Verification items for the finished model (mm, model axes). A direction names the side the tool comes from. Round coordinates to 2 decimals unless told otherwise and drop trailing zeros. Write each loop counter-clockwise with the first axis right and the second up, starting at its lowest first coordinate (ties: lowest second). Pieces come first, ordered by that corner, then holes. Notation, with made-up numbers: (37.25, 61.25) -> (51.25, 61.25) arc R7 cw to (51.25, 66.25) -> close; hole circle Ø7 at (-9, 70.5). An arc over 180 degrees is marked (long way). Answer as a JSON object with one key per item and string values. Group by question number.
(1) Sectioned sample at A-A on y = 16. Record the cut outline in (x, z) (1 decimal).
(2) Scan lines: L1, parallel to X at y = 6, z = 34 (3 decimals); L2, parallel to X at y = 23, z = -20.5 (3 decimals); L3, parallel to Z at x = 10, y = 2 (1 decimal). Record each from-to range of solid material in increasing order. Write a range as from..to.
(3) Sectioned sample at D-D on y = 20. Count the separate pieces of the cut face and the enclosed holes in it, and give its area (3 significant figures).
(4) Draft check along Z on faces 1 (the face through (-19.49, 6.37, 27.18)), 2 (the face through (-24.6, 17.26, 25.98)), 3 (the face through (28.575, 16, 5)). Enter one of: released by +Z, released by -Z, zero draft, split by the parting line, or undercut.
(5) Set-up check for faces 4 (the face through (16.71, 27.546, 33.404)), 5 (the face through (-7, 31.75, 19)), 6 (the face through (26.1, 3.175, 4.1)): record each of +Z, -Z, +X, -X, +Y, -Y from which the full face is reachable in a straight line by a thin tool's end or side.
(6) Gauge pin test, flat ends, axial feed: pin 1 Ø2 at (x, z) = (16.5, -4.5) entering from -Y; pin 2 Ø18 at (x, z) = (0, 0) entering from +Y; pin 3 Ø15.5 at (x, z) = (9, 11.5) entering from -Y; pin 4 Ø3 at (x, y) = (19, 7) entering from +Z. Record the tip position at first contact, or that the pin passes through.
```python
from build123d import *

# Parameters (mm, degrees)
SKETCH1_R                         = 2.5527
BOSS_EXTRUDE1_DEPTH               = 31.75
SKETCH2_R                         = 19.05
CUT_EXTRUDE1_DEPTH                = 1.524
SKETCH3_R                         = 11.1125
CUT_EXTRUDE2_DEPTH                = 57.407018189
CUT_EXTRUDE3_DEPTH                = 23.876
SKETCH5_R                         = 26.19375
CUT_EXTRUDE4_DEPTH                = 17.526
CUT_EXTRUDE5_DEPTH                = 3.175
F_1_4_20_TAPPED_HOLE1_D           = 5.1054
F_1_4_20_TAPPED_HOLE1_DEPTH       = 9.652
F_1_4_20_TAPPED_HOLE1_CBORE_D     = 6.35
F_1_4_20_TAPPED_HOLE1_CBORE_DEPTH = 9.525
F_1_4_20_TAPPED_HOLE1_TIP         = 1.533816902


with BuildPart() as part:
    # Sketch1 → Boss-Extrude1 (new body)
    with BuildSketch(Plane(origin=(0, 0, 0), x_dir=(1, 0, 0), z_dir=(0, 1, 0))):
        Polygon((28.575, 28.575), (-28.575, 28.575), (-28.575, -28.575), (-28.575, -38.1), (28.575, -38.1), (28.575, -28.575), align=None)
        with Locations(Location((23.622, -23.622, 0), (0, 0, 270))):
            Circle(SKETCH1_R, mode=Mode.SUBTRACT)
        with Locations(Location((23.622, 23.622, 0), (0, 0, 270))):
            Circle(SKETCH1_R, mode=Mode.SUBTRACT)
        with Locations(Location((-23.622, 23.622, 0), (0, 0, 270))):
            Circle(SKETCH1_R, mode=Mode.SUBTRACT)
        with Locations(Location((-23.622, -23.622, 0), (0, 0, 270))):
            Circle(SKETCH1_R, mode=Mode.SUBTRACT)
    extrude(amount=BOSS_EXTRUDE1_DEPTH)

    # Sketch2 → Cut-Extrude1 (cut)
    with BuildSketch(Plane(origin=(0, 31.75, 0), x_dir=(1, 0, 0), z_dir=(0, 1, 0))):
        with Locations(Location((0, 0, 0), (0, 0, 270))):
            Circle(SKETCH2_R)
    extrude(amount=-CUT_EXTRUDE1_DEPTH, mode=Mode.SUBTRACT)

    # Sketch3 → Cut-Extrude2 (cut, through all)
    with BuildSketch(Plane(origin=(0, 30.226, 0), x_dir=(1, 0, 0), z_dir=(0, 1, 0))):
        with Locations(Location((0, 0, 0), (0, 0, 270))):
            Circle(SKETCH3_R)
    extrude(amount=-CUT_EXTRUDE2_DEPTH, mode=Mode.SUBTRACT)

    # Sketch4 → Cut-Extrude3 (cut)
    with BuildSketch(Plane.XZ):
        with BuildLine():
            ThreePointArc((0, 20.955), (1.652808564, 21.41912397), (2.822399445, 22.675803874))
            ThreePointArc((2.822399445, 22.675803874), (7.210100154, 24.555346085), (9.885111639, 20.602004462))
            ThreePointArc((9.885111639, 20.602004462), (10.189621648, 18.912489483), (11.32912833, 17.62846778))
            ThreePointArc((11.32912833, 17.62846778), (12.970483736, 17.125337937), (14.633818648, 17.550195776))
            ThreePointArc((14.633818648, 17.550195776), (19.341144607, 16.759197203), (19.454169622, 11.9872142))
            ThreePointArc((19.454169622, 11.9872142), (18.796918984, 10.401273215), (19.061338463, 8.705021597))
            ThreePointArc((19.061338463, 8.705021597), (20.170121967, 7.39437811), (21.799103827, 6.852524522))
            ThreePointArc((21.799103827, 6.852524522), (25.331512305, 3.642121623), (22.846666207, -0.433431873))
            ThreePointArc((22.846666207, -0.433431873), (21.436327355, -1.412273807), (20.741708315, -2.982207436))
            ThreePointArc((20.741708315, -2.982207436), (20.965888988, -4.68424452), (22.043327566, -6.02077485))
            ThreePointArc((22.043327566, -6.02077485), (23.27930383, -10.631301837), (18.985507698, -12.716466389))
            ThreePointArc((18.985507698, -12.716466389), (17.269853253, -12.777433874), (15.836732331, -13.72260668))
            ThreePointArc((15.836732331, -13.72260668), (15.105134394, -15.275652613), (15.288950554, -16.982520747))
            ThreePointArc((15.288950554, -16.982520747), (13.836080873, -21.529362082), (9.09658464, -20.962112676))
            ThreePointArc((9.09658464, -20.962112676), (7.620322766, -20.085848967), (5.903705729, -20.106175262))
            ThreePointArc((5.903705729, -20.106175262), (4.448606357, -21.017148933), (3.680439768, -22.552436301))
            ThreePointArc((3.680439768, -22.552436301), (0, -25.592001984), (-3.680439768, -22.552436301))
            ThreePointArc((-3.680439768, -22.552436301), (-4.448606357, -21.017148933), (-5.903705729, -20.106175262))
            ThreePointArc((-5.903705729, -20.106175262), (-7.620322766, -20.085848967), (-9.09658464, -20.962112676))
            ThreePointArc((-9.09658464, -20.962112676), (-13.836080873, -21.529362082), (-15.288950554, -16.982520747))
            ThreePointArc((-15.288950554, -16.982520747), (-15.105134394, -15.275652613), (-15.836732331, -13.72260668))
            ThreePointArc((-15.836732331, -13.72260668), (-17.269853253, -12.777433874), (-18.985507698, -12.716466389))
            ThreePointArc((-18.985507698, -12.716466389), (-23.27930383, -10.631301837), (-22.043327566, -6.02077485))
            ThreePointArc((-22.043327566, -6.02077485), (-20.965888988, -4.68424452), (-20.741708315, -2.982207436))
            ThreePointArc((-20.741708315, -2.982207436), (-21.436327355, -1.412273807), (-22.846666207, -0.433431873))
            ThreePointArc((-22.846666207, -0.433431873), (-25.331512305, 3.642121623), (-21.799103827, 6.852524522))
            ThreePointArc((-21.799103827, 6.852524522), (-20.170121967, 7.39437811), (-19.061338463, 8.705021597))
            ThreePointArc((-19.061338463, 8.705021597), (-18.796918984, 10.401273215), (-19.454169622, 11.9872142))
            ThreePointArc((-19.454169622, 11.9872142), (-19.341144607, 16.759197203), (-14.633818648, 17.550195776))
            ThreePointArc((-14.633818648, 17.550195776), (-12.970483736, 17.125337937), (-11.32912833, 17.62846778))
            ThreePointArc((-11.32912833, 17.62846778), (-10.189621648, 18.912489483), (-9.885111639, 20.602004462))
            ThreePointArc((-9.885111639, 20.602004462), (-7.210100154, 24.555346085), (-2.822399445, 22.675803874))
            ThreePointArc((-2.822399445, 22.675803874), (-1.652808564, 21.41912397), (0, 20.955))
        make_face()
    extrude(amount=-CUT_EXTRUDE3_DEPTH, mode=Mode.SUBTRACT)

    # Sketch5 → Cut-Extrude4 (cut)
    with BuildSketch(Plane.XZ):
        with Locations(Location((0, 0, 0), (0, 0, 270))):
            Circle(SKETCH5_R)
    extrude(amount=-CUT_EXTRUDE4_DEPTH, mode=Mode.SUBTRACT)

    # Sketch7 → Cut-Extrude5 (cut)
    with BuildSketch(Plane.XZ):
        with BuildLine():
            Line((-23.8125, 26.9875), (23.8125, 26.9875))
            ThreePointArc((23.8125, 26.9875), (26.05756403, 26.05756403), (26.9875, 23.8125))
            Line((26.9875, 23.8125), (26.9875, -23.8125))
            ThreePointArc((26.9875, -23.8125), (26.05756403, -26.05756403), (23.8125, -26.9875))
            Line((23.8125, -26.9875), (-23.8125, -26.9875))
            ThreePointArc((-23.8125, -26.9875), (-26.05756403, -26.05756403), (-26.9875, -23.8125))
            Line((-26.9875, -23.8125), (-26.9875, 23.8125))
            ThreePointArc((-26.9875, 23.8125), (-26.05756403, 26.05756403), (-23.8125, 26.9875))
        make_face()
    extrude(amount=-CUT_EXTRUDE5_DEPTH, mode=Mode.SUBTRACT)

    # 1/4-20 Tapped Hole1
    with Locations(Plane.XY.offset(38.1)):
        with Locations((-19.05, 25.4), (19.05, 25.4), (19.05, 6.35), (-19.05, 6.35)):
            CounterBoreHole(F_1_4_20_TAPPED_HOLE1_D / 2, F_1_4_20_TAPPED_HOLE1_CBORE_D / 2, F_1_4_20_TAPPED_HOLE1_CBORE_DEPTH, depth=F_1_4_20_TAPPED_HOLE1_DEPTH)
            with Locations((0, 0, -(F_1_4_20_TAPPED_HOLE1_DEPTH + F_1_4_20_TAPPED_HOLE1_TIP / 2))):  # 118° drill point
                Cone(0, F_1_4_20_TAPPED_HOLE1_D / 2, F_1_4_20_TAPPED_HOLE1_TIP, mode=Mode.SUBTRACT)


solid = part.part
```
Computed values:
{
 "1": {"outline": "(-28.6, -28.6) -> (28.6, -28.6) -> (28.6, 38.1) -> (-28.6, 38.1) -> close; hole circle Ø5.1 at (-23.6, -23.6); hole circle Ø52.4 at (0, 0); hole circle Ø5.1 at (-23.6, 23.6); hole circle Ø5.1 at (23.6, -23.6); hole circle Ø5.1 at (23.6, 23.6)"},
 "2": {"L1": "-28.575..-22.206, -15.894..15.894, 22.206..28.575", "L2": "-28.575..-14.898, -8.543..-5.053, 5.053..8.543, 14.898..28.575", "L3": "-28.6..-27, 27..38.1"},
 "3": {"separate pieces": "1", "enclosed holes": "5", "area": "2,000 mm2"},
 "4": {"face 1": "released by +Z", "face 2": "undercut", "face 3": "zero draft"},
 "5": {"face 4": "+Z", "face 5": "+Z, -Z, +X, -X, +Y", "face 6": "-Y"},
 "6": {"pin 1": "y = 23.88", "pin 2": "through", "pin 3": "y = 17.53", "pin 4": "z = 28.21"}
}
